```python
from build123d import *

# Parameters (mm, degrees)
SKETCH_1_R          = 17.5
EXTRUDE_1_DEPTH     = 15
SKETCH_2_R          = 3
CUT_EXTRUDE_1_DEPTH = 16
SKETCH_3_R          = 1.5
CUT_EXTRUDE_2_DEPTH = 5
SKETCH_4_R          = 1.5
CUT_EXTRUDE_3_DEPTH = 5


with BuildPart() as part:
    # 草图1 → 凸台-拉伸1 (new body)
    with BuildSketch(Plane(origin=(0, 0, 0), x_dir=(1, 0, 0), z_dir=(0, 1, 0))):
        Circle(SKETCH_1_R)
    extrude(amount=EXTRUDE_1_DEPTH)

    # 草图2 → 切除-拉伸1 (cut, through all)
    with BuildSketch(Plane(origin=(0, 0, 0), x_dir=(-1, 0, 0), z_dir=(0, -1, 0))):
        Circle(SKETCH_2_R)
    extrude(amount=-CUT_EXTRUDE_1_DEPTH, mode=Mode.SUBTRACT)

    # 草图3 → 切除-拉伸2 (cut)
    with BuildSketch(Plane(origin=(0, 15, 0), x_dir=(1, 0, 0), z_dir=(0, 1, 0))):
        with Locations((0, 8)):
            Circle(SKETCH_3_R)
        with Locations((8, 0)):
            Circle(SKETCH_3_R)
        with Locations((0, -8)):
            Circle(SKETCH_3_R)
        with Locations((-8, 0)):
            Circle(SKETCH_3_R)
    extrude(amount=-CUT_EXTRUDE_2_DEPTH, mode=Mode.SUBTRACT)

    # 草图4 → 切除-拉伸3 (cut)
    with BuildSketch(Plane.XZ):
        with Locations((0, 9.5)):
            Circle(SKETCH_4_R)
        with Locations((9.5, 0)):
            Circle(SKETCH_4_R)
        with Locations((0, -9.5)):
            Circle(SKETCH_4_R)
        with Locations((-9.5, 0)):
            Circle(SKETCH_4_R)
    extrude(amount=-CUT_EXTRUDE_3_DEPTH, mode=Mode.SUBTRACT)


solid = part.part
```
Could you check a few things on this model? Use its own coordinates, in mm. A direction names the side the tool comes from. Coordinates: 2 decimals unless noted, no trailing zeros. Loops run counter-clockwise (first coordinate to the right, second up) from the corner with the lowest first, then second, coordinate; pieces in that order, holes last. Notation, with made-up numbers: M 53,8 L 61,8 A12 cw 61,28 Z; hole C -20,30.25 d5. An arc over 180 degrees is marked long. Put each result on its own line as item: value. Start each with the question number.
(1) Suppose I cut it at A-A on z = 0. Please give me the cut outline in (x, y), then the cut area to 3 significant figures.
(2) Suppose I cut it at D-D on y = 9.25. Please give me the cut outline in (x, z).
(3) Thinking about a two-plate mould opening in X: for faces 4 (the face through (0, 15, 4)), 5 (the face through (-13.887, 7.395, 10.648)), 6 (the face through (-9.5, 12.54, -0.07)), which applies, pulls with the +X half, pulls with the -X half, needs draft (parallel to the pull), parting line crosses it, or undercut?
(4) Suppose I cut it at C-C on y = 2. Please give me the cut outline in (x, z), then the cut area to 3 significant figures.
(5) For faces 1 (the face through (0, 5, -9)), 2 (the face through (0, 0, 4)), 3 (the face through (0, 10, 8)), which set-ups out of +Z, -Z, +X, -X, +Y, -Y let a thin tool reach every point of the face, with its end or its side?
(6) Suppose I cut it at B-B on x = 0. Please give me the cut outline in (y, z).
(7) I need wall thicknesses on line 1 (Z direction, x = 0, y = 13.2); line 2 (Z direction, x = 9.5, y = 2.95). Which ranges of each line are inside material? Lowest first, please. Write a range as from..to.
(8) Will these pins go through, and if not, where does the flat tip stop? P1, Ø9.5, axis at x = 0, z = 0, coming from the +Y side; P2, Ø0.9, axis at x = 0, z = -8.5, coming from the +Y side; P3, Ø3, axis at x = -6.5, y = 2.5, coming from the +Z side; P4, Ø0.9, axis at x = -10, z = -0.5, coming from the -Y side.
Solutions:
1. outline: M -17.5,0 L -11,0 L -11,5 L -8,5 L -8,0 L -3,0 L -3,15 L -6.5,15 L -6.5,10 L -9.5,10 L -9.5,15 L -17.5,15 Z; M 3,0 L 8,0 L 8,5 L 11,5 L 11,0 L 17.5,0 L 17.5,15 L 9.5,15 L 9.5,10 L 6.5,10 L 6.5,15 L 3,15 Z
1. area: 375 mm2
2. outline: C 0,0 d35; hole C 0,0 d6
3. face 4: needs draft
3. face 5: parting line crosses it
3. face 6: undercut
4. outline: C 0,0 d35; hole C -9.5,0 d3; hole C 0,0 d6; hole C 0,-9.5 d3; hole C 0,9.5 d3; hole C 9.5,0 d3
4. area: 906 mm2
5. face 1: -Y
5. face 2: +Z, -Z, +X, -X, -Y
5. face 3: +Y
6. outline: M 0,-17.5 L 15,-17.5 L 15,-9.5 L 10,-9.5 L 10,-6.5 L 15,-6.5 L 15,-3 L 0,-3 L 0,-8 L 5,-8 L 5,-11 L 0,-11 Z; M 0,3 L 15,3 L 15,6.5 L 10,6.5 L 10,9.5 L 15,9.5 L 15,17.5 L 0,17.5 L 0,11 L 5,11 L 5,8 L 0,8 Z
7. line 1: z = -17.5..-9.5, -6.5..-3, 3..6.5, 9.5..17.5
7. line 2: z = -14.7..-1.5, 1.5..14.7
8. P1: stops at y = 15
8. P2: stops at y = 10
8. P3: stops at z = 16.77
8. P4: stops at y = 5
